Autodesk Inventor part; units mm, degrees
ref_plane "YZ Plane" through (0, 0, 0) normal (1, 0, 0) x (0, 1, 0)
ref_plane "XZ Plane" through (0, 0, 0) normal (0, 1, 0) x (-1, 0, 0)
ref_plane "XY Plane" through (0, 0, 0) normal (0, 0, 1) x (1, 0, 0)
sketch "Sketch1" plane through (0, 0, 0) normal (0, 1, 0) x (-1, 0, 0)
  line L0 (67.5641, 73.7231) -> (97.6281, -21.6506)
  line L1 (97.6281, -21.6506) -> (30.0641, -95.3738)
  line L2 (30.0641, -95.3738) -> (-67.5641, -73.7231)
  line L3 (-67.5641, -73.7231) -> (-97.6281, 21.6506)
  line L4 (-97.6281, 21.6506) -> (-30.0641, 95.3738)
  line L5 (-30.0641, 95.3738) -> (67.5641, 73.7231)
  point P0 (0, 0)
  point P1 (0, 0)
  dimension "d0" = 100
  dimension "d17" = 21.6506
extrude "Extrusion1" add sketch "Sketch1" along normal blind 8
sketch "Sketch2" plane through (67.5641, 0, -73.7231) normal (0.9537, 0, -0.3006) x (-0.3006, 0, -0.9537)
  line L0 (0, 0) -> (0, 8)
  line L1 (0, 4) -> (-5, 4)
  line L2 (-100, 0) -> (-100, 8)
  line L3 (-100, 4) -> (-95, 4)
  circle A0 centre (-95, 4) radius 1
  circle A1 centre (-5, 4) radius 1
  point P0 (-50, 0)
  dimension "d4" = 5
  dimension "d5" = 5
  dimension "d6" = 2
  dimension "d7" = 2
extrude "Extrusion2" cut sketch "Sketch2" against normal blind 10
sketch "Sketch3" plane through (0, 8, 0) normal (0, 1, 0) x (1, 0, 0)
  circle A0 centre (0, 0) radius 0.5
  dimension "d10" = 1
extrude "Extrusion3" cut sketch "Sketch3" against normal blind 5
pattern_circular "Circular Pattern1" count 3 over 360 about axis through (0, 8, 0) along (0, -1, 0) of "Extrusion2"
sketch "Sketch4" plane through (0, 8, 0) normal (0, 1, 0) x (1, 0, 0)
  line L0 (0, 0) -> (0, 10.5)
  line L1 (0, 10.5) -> (-6.25, 10.5)
  circle A0 centre (-6.25, 10.5) radius 1.5
  circle A1 centre (6.25, 10.5) radius 1.5
  circle A2 centre (-6.25, -10.5) radius 1.5
  circle A3 centre (6.25, -10.5) radius 1.5
  dimension "d18" = 10.5
  dimension "d19" = 6.25
  dimension "d20" = 3
  dimension "d23" = 12.5
  dimension "d26" = 21
extrude "Extrusion4" cut sketch "Sketch4" against normal blind 8
sketch "Sketch5" plane through (0, 8, 0) normal (0, 1, 0) x (1, 0, 0)
  line L0 (-67.5641, -73.7231) -> (30.0641, -95.3738)
  line L1 (30.0641, -95.3738) -> (25.1827, -94.2912)
  line L2 (25.1827, -94.2912) -> (26.0487, -90.3861)
  line L3 (26.0487, -90.3861) -> (23.852, -89.899)
  line L4 (26.0487, -90.3861) -> (28.2453, -90.8732)
  line L5 (23.852, -89.899) -> (24.3933, -87.4583)
  line L6 (24.3933, -87.4583) -> (28.7866, -88.4325)
  line L7 (28.7866, -88.4325) -> (28.2453, -90.8732)
  point P0 (0, 0)
  dimension "d31" = 5
  dimension "d32" = 4
  dimension "d33" = 2.25
  dimension "d34" = 90
  dimension "d35" = 2.25
  dimension "d36" = 90
  dimension "d37" = 2.5
  dimension "d38" = 90
  dimension "d39" = 90
extrude "Extrusion5" cut sketch "Sketch5" against normal blind 8
pattern_linear "Rectangular Pattern1" count 2 spacing 65 along (-0.9763, 0, -0.2165) of "Extrusion5"
pattern_circular "Circular Pattern2" count 3 over 360 about axis through (0, 8, 0) along (0, -1, 0) of "Extrusion5", "Rectangular Pattern1"
sketch "Sketch6" plane through (0, 8, 0) normal (0, 1, 0) x (1, 0, 0)
  line L0 (-97.6281, 21.6506) -> (-30.0641, 95.3738)
  line L1 (-97.6281, 21.6506) -> (-30.0641, 95.3738)
  line L2 (-30.0641, 95.3738) -> (67.5641, 73.7231)
  line L3 (-30.0641, 95.3738) -> (67.5641, 73.7231)
  line L4 (67.5641, 73.7231) -> (97.6281, -21.6506)
  line L5 (67.5641, 73.7231) -> (97.6281, -21.6506)
  line L6 (97.6281, -21.6506) -> (30.0641, -95.3738)
  line L7 (97.6281, -21.6506) -> (30.0641, -95.3738)
  line L8 (30.0641, -95.3738) -> (-67.5641, -73.7231)
  line L9 (-61.7064, -75.0222) -> (-63.6589, -74.5891)
  line L10 (-67.5641, -73.7231) -> (-97.6281, 21.6506)
  line L11 (-80.7184, 17.9006) -> (-24.8568, 78.8545)
  line L12 (-24.8568, 78.8545) -> (55.8616, 60.9539)
  line L13 (55.8616, 60.9539) -> (80.7184, -17.9006)
  line L14 (80.7184, -17.9006) -> (24.8568, -78.8545)
  line L15 (24.8568, -78.8545) -> (-55.8616, -60.9539)
  line L16 (-55.8616, -60.9539) -> (-80.7184, 17.9006)
  line L17 (0, 0) -> (30, 0) construction
  line L18 (8.8449, -28.0592) -> (28.7224, -6.3697)
  line L19 (28.7224, -6.3697) -> (19.8775, 21.6895)
  line L20 (19.8775, 21.6895) -> (-8.8449, 28.0592)
  line L21 (-8.8449, 28.0592) -> (-28.7224, 6.3697)
  line L22 (-28.7224, 6.3697) -> (-19.8775, -21.6895)
  line L23 (-19.8775, -21.6895) -> (8.8449, -28.0592)
  line L24 (28.7224, -6.3697) -> (19.8775, 21.6895)
  line L25 (-8.8449, 28.0592) -> (-28.7224, 6.3697)
  line L26 (-19.8775, -21.6895) -> (8.8449, -28.0592)
  line L27 (0, 0) -> (8.8449, -28.0592)
  line L28 (-8.8449, 28.0592) -> (-28.7224, 6.3697)
  line L29 (-28.7224, 6.3697) -> (-62.7264, 37.5328)
  line L30 (-62.7264, 37.5328) -> (-42.8489, 59.2223)
  line L31 (-42.8489, 59.2223) -> (-8.8449, 28.0592)
  line L32 (-19.8775, -21.6895) -> (8.8449, -28.0592)
  line L33 (8.8449, -28.0592) -> (-1.1412, -73.089)
  line L34 (-1.1412, -73.089) -> (-29.8636, -66.7194)
  line L35 (-29.8636, -66.7194) -> (-19.8775, -21.6895)
  line L36 (28.7224, -6.3697) -> (19.8775, 21.6895)
  line L37 (19.8775, 21.6895) -> (63.8676, 35.5562)
  line L38 (63.8676, 35.5562) -> (72.7125, 7.497)
  line L39 (72.7125, 7.497) -> (28.7224, -6.3697)
  dimension "d50" = 15
  dimension "d53" = 28.7224
fillet "Fillet2" radius 2 6 edges at (-97.6281, 4, -21.6506) (-67.5641, 4, 73.7231) (30.0641, 4, 95.3738) (97.6281, 4, 21.6506) (67.5641, 4, -73.7231) (-30.0641, 4, -95.3738)
extrude "Extrusion7" cut sketch "Sketch6" against normal blind 10 contours L11 L29 L22 L35 L15 L16 | L11 L12 L13 L37 L20 L31 | L33 L18 L39 L13 L14 L15
properties part number "Hex_Servo_Top"
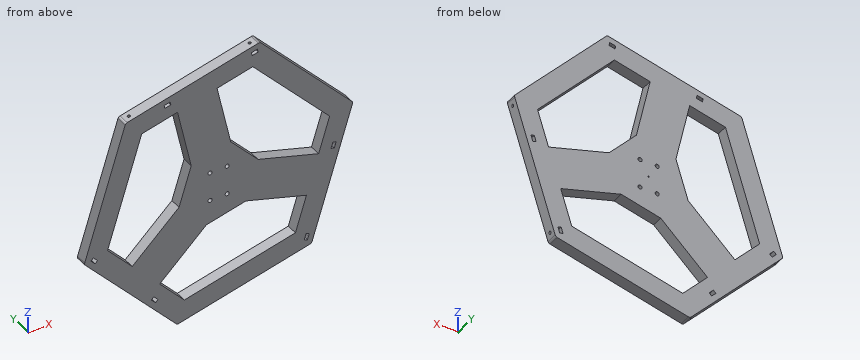
CAD build for the part. Positions are in the model's coordinates, mm. Coordinates: 2 decimals unless noted, no trailing zeros. Order: outer loops, then holes, each group sorted by start corner. A loop starts at its lowest first (then second) coordinate and runs counter-clockwise, first axis right, second up. Notation, with made-up numbers: (12, 6) - (71, 6) arc R22 ccw to (71, 34) - close; hole circle Ø3 at (34, 31). An arc over 180 degrees is marked (long way). Answer in a Markdown table with one row per item.
1. Flat gauge pins, fed straight in: P1, Ø4, axis at x = -32, z = -29, coming from the -Y side; P2, Ø1.8, axis at x = 6.25, z = -10.5, coming from the +Y side; P3, Ø0.5, axis at x = 0, z = 0, coming from the +Y side; P4, Ø2, axis at y = 1.5, z = -45.5, coming from the -X side. Where does each tip first touch, or does it go through?
Answer:
| item | result |
|---|---|
| P1 | y = 0 |
| P2 | through |
| P3 | y = 3 |
| P4 | x = -76.69 |
2. Slice it at B-B, the plane z = 36.5. List the corners of the cut face in (x, y), then the cut area to 3 significant figures.
Answer:
| item | result |
|---|---|
| outline | (-79.3, 0) - (-63.57, 0) - (-63.57, 8) - (-79.3, 8) - close; (-23.16, 0) - (6.97, 0) - (6.97, 8) - (-23.16, 8) - close; (63.67, 0) - (84.02, 0) - (84.02, 8) - (63.67, 8) - close |
| area | 530 mm² |
3. Slice it at D-D, the plane y = 6.5. Give the number of separate pieces and of enclosed holes in the cut face, then the cut area to 3 significant figures.
Answer:
| item | result |
|---|---|
| separate pieces | 1 |
| enclosed holes | 14 |
| area | 14,400 mm² |
4. Slice it at C-C, the plane x = -77. List the corners of the cut face in (y, z).
Answer:
| item | result |
|---|---|
| outline | (0, -44.16) - (8, -44.16) - (8, -21.96) - (0, -21.96) - close; (0, -6.1) - (8, -6.1) - (8, 43.79) - (0, 43.79) - close |
5. Drill centre lines: L1, parallel to Z at x = -6.25, y = 2.75; L2, parallel to Z at x = -45, y = 3.25; L3, parallel to X at y = 3, z = 10.5. Where is each one in solid material? Low to high. Write a range as from..to.
Answer:
| item | result |
|---|---|
| L1 | -90.09..-74.73, -27.48..-12, -9..9, 12..87.32 |
| L2 | -79.08..-71.42, -69.46..-21.29, 63.36..78.73 |
| L3 | -87.49..-71.77, -23.4..-7.75, -4.75..4.75, 7.75..24.94, 78.39..94.11 |
6. Slice it at A-A, the plane x = -17. List the corners of the cut face in (y, z).
Answer:
| item | result |
|---|---|
| outline | (0, -92.48) - (8, -92.48) - (8, -77.11) - (0, -77.11) - close; (0, -35.53) - (8, -35.53) - (8, 84.94) - (0, 84.94) - close |
